Here's the drawing with two shaded views (mm, measured from the low corner). I have some questions. A direction names the side the tool comes from. Give positions to 0.01 mm unless a question says otherwise; leave off trailing zeros. Order: outer loops, then holes, each group sorted by start corner. A loop starts at its lowest first (then second) coordinate and runs counter-clockwise, first axis right, second up. Notation, with made-up numbers: (-25.75, 34.25) - (-20.75, 34.25) arc R34 ccw to (-20.75, 72.25) - close; hole circle Ø7 at (29.5, 86.25). An arc over 180 degrees is marked (long way). Use one line per item in the form item = value. Start each with the question number.
1) Which directions (+Z, -Z, +X, -X, +Y, -Y) give clear straight access to the entire face, cutting with the end or side of a thin tool? Please do the marked faces 1 and 2.
2) We'd pull the mould along Z, two halves only. Please class the marked faces 3, 4, 5 and 6: released by +Z, released by -Z, zero draft, split by the parting line, or undercut.
3) Suppose I cut it at A-A, the plane x = 29. Write out the boundary of the cut face in (y, z), and give its area (3 significant figures).
4) Please list where these lines run through material, in increasing order: probe 1 along Z at (x, y) = (33, 42); probe 2 along X at (y, z) = (43.5, 30).
5) Suppose I cut it at B-B, the plane z = 14. Write out the boundary of the cut face in (x, y), and give its area (3 significant figures).
6) Suppose I cut it at C-C, the plane y = 25.5. Write out the boundary of the cut face in (x, z).
7) Suppose I cut it at D-D, the plane y = 89. Write out the boundary of the cut face in (x, z).
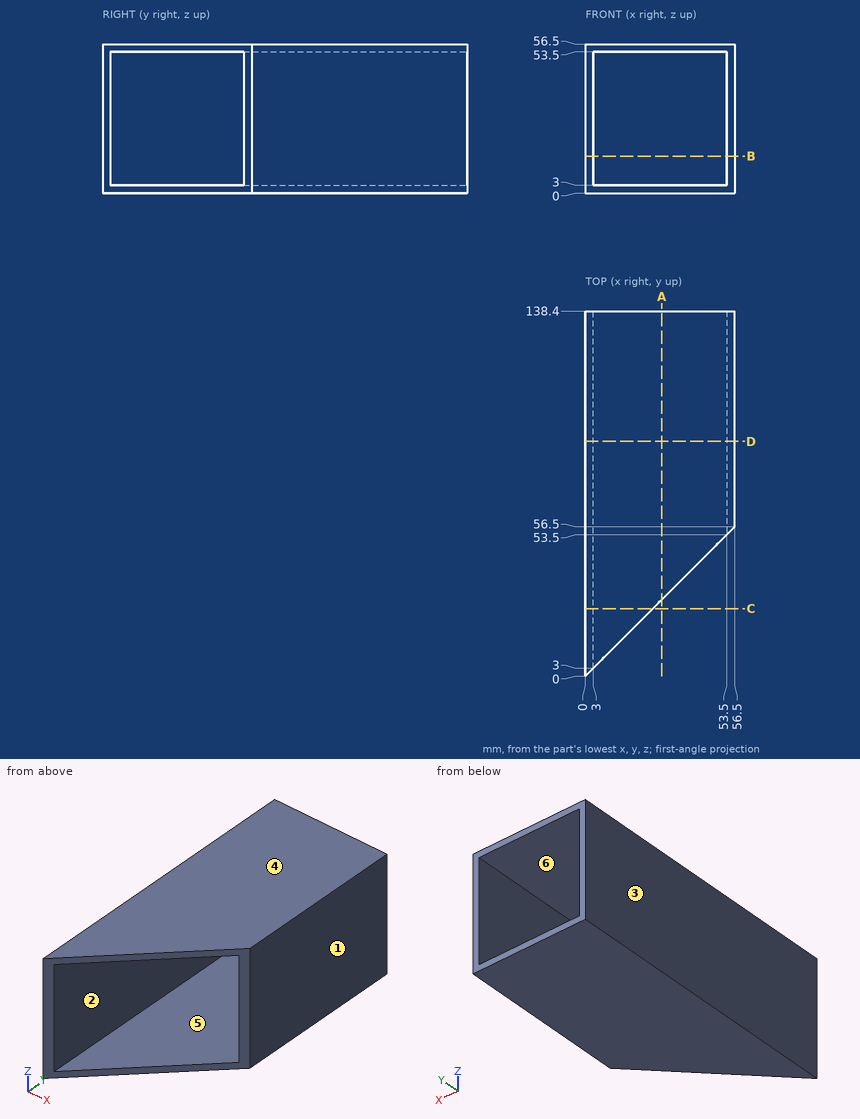
Result sheet:
q1.face_1 = +Z, -Z, +X, +Y, -Y
q1.face_2 = +Y, -Y
q2.face_3 = zero draft
q2.face_4 = released by +Z
q2.face_5 = undercut
q2.face_6 = undercut
q3.outline = (29, 0) - (138.4, 0) - (138.4, 3) - (29, 3) - close; (29, 53.5) - (138.4, 53.5) - (138.4, 56.5) - (29, 56.5) - close
q3.area = 656 mm²
q4.probe_1 = 0 to 3, 53.5 to 56.5
q4.probe_2 = 0 to 3
q5.outline = (0, 0) - (3, 3) - (3, 138.4) - (0, 138.4) - close; (53.5, 53.5) - (56.5, 56.5) - (56.5, 138.4) - (53.5, 138.4) - close
q5.area = 661 mm²
q6.outline = (0, 0) - (25.5, 0) - (25.5, 3) - (3, 3) - (3, 53.5) - (25.5, 53.5) - (25.5, 56.5) - (0, 56.5) - close
q7.outline = (0, 0) - (56.5, 0) - (56.5, 56.5) - (0, 56.5) - close; hole (3, 3) - (53.5, 3) - (53.5, 53.5) - (3, 53.5) - close
